The figure shows three views and two pictorial views of one solid part (mm, origin at its lowest corner). Answer the questions. A direction names the side the tool comes from. Coordinates: 2 decimals unless noted, no trailing zeros. Order: outer loops, then holes, each group sorted by start corner. A loop starts at its lowest first (then second) coordinate and runs counter-clockwise, first axis right, second up. Notation, with made-up numbers: (-3, 7) -> (1, 7) arc R19 ccw to (1, 31) -> close; hole circle Ø10 at (47.25, 48). An arc over 180 degrees is marked (long way). Use one line per item in the form item = value.
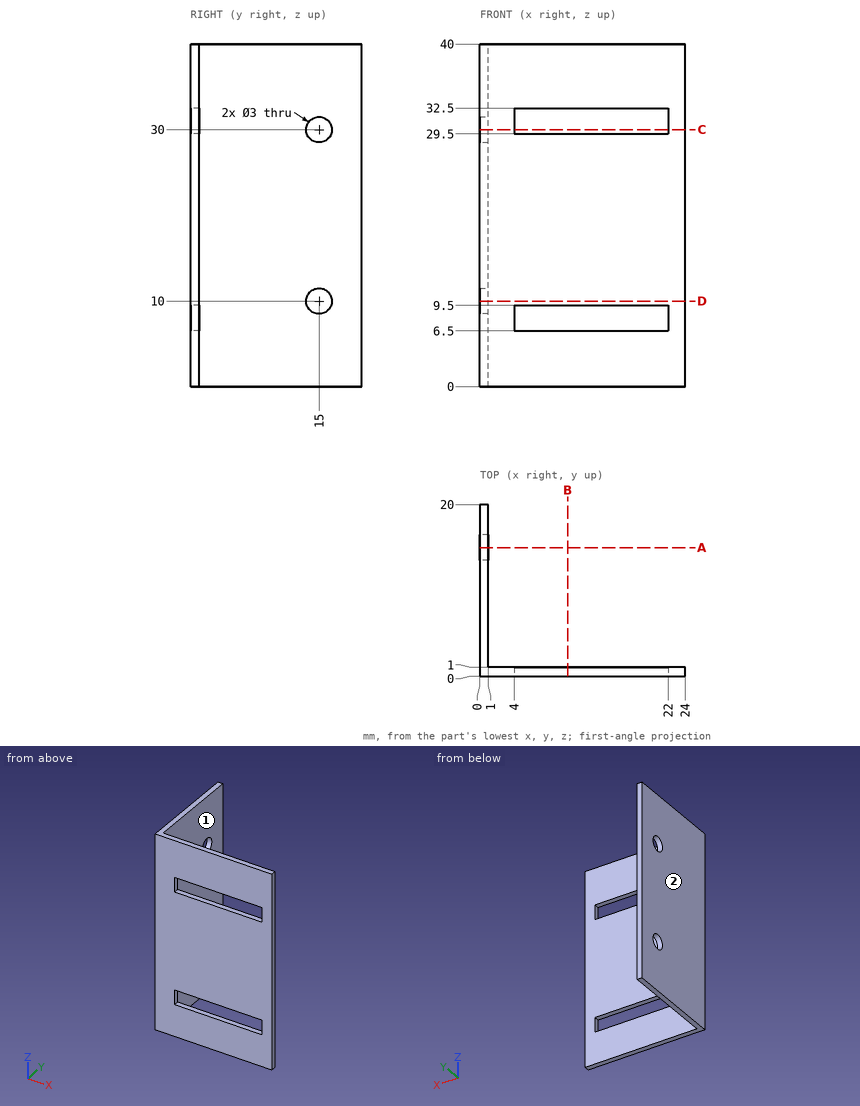
(1) Section D-D on z = 10 is taken. Write down the section's boundary in (x, y).
Data:
outline = (0, 0) -> (24, 0) -> (24, 1) -> (1, 1) -> (1, 13.5) -> (0, 13.5) -> close; (0, 16.5) -> (1, 16.5) -> (1, 20) -> (0, 20) -> close
(2) Section A-A on y = 15 is taken. Write down the section's boundary in (x, z), plus the area to 3 significant figures.
Data:
outline = (0, 0) -> (1, 0) -> (1, 8.5) -> (0, 8.5) -> close; (0, 11.5) -> (1, 11.5) -> (1, 28.5) -> (0, 28.5) -> close; (0, 31.5) -> (1, 31.5) -> (1, 40) -> (0, 40) -> close
area = 34.0 mm²
(3) Each of these flat-tipped pins is pushed along its axis until it touches: P1, Ø6, axis at x = 21.5, z = 15.5, coming from the +Y side; P2, Ø2, axis at y = 10, z = 4.5, coming from the +X side; P3, Ø2.5, axis at y = 15, z = 10, coming from the -X side. Where does it stop, or does it pass through?
Data:
P1 = 1
P2 = 1
P3 = through
(4) Section C-C on z = 30 is taken. Write down the section's boundary in (x, y).
Data:
outline = (0, 0) -> (4, 0) -> (4, 1) -> (1, 1) -> (1, 13.5) -> (0, 13.5) -> close; (0, 16.5) -> (1, 16.5) -> (1, 20) -> (0, 20) -> close; (22, 0) -> (24, 0) -> (24, 1) -> (22, 1) -> close
(5) Straight lines are drawn through the part: line 1 along Y through (x, z) = (0.6, 30); line 2 along X through (y, z) = (8.75, 30). For each, find the intervals that lie inside material, in ascending order.
Data:
line_1 = 0 to 13.5, 16.5 to 20
line_2 = 0 to 1
(6) Which of the six approach directions +Z, -Z, +X, -X, +Y, -Y give full straight-line access (tool end or side, diameter ignored) to the marked faces 1 and 2?
Data:
face_1 = +Z, -Z, +X, +Y
face_2 = +Z, -Z, -X, +Y, -Y
(7) Section B-B on x = 10.25 is taken. Write down the section's boundary in (y, z), plus the area to 3 significant figures.
Data:
outline = (0, 0) -> (1, 0) -> (1, 6.5) -> (0, 6.5) -> close; (0, 9.5) -> (1, 9.5) -> (1, 29.5) -> (0, 29.5) -> close; (0, 32.5) -> (1, 32.5) -> (1, 40) -> (0, 40) -> close
area = 34.0 mm²
